```python
from build123d import *

# Parameters (mm, degrees)
SKETCH1_R           = 1.65
SKETCH1_R_2         = 7
BOSS_EXTRUDE1_DEPTH = 3.175


with BuildPart() as part:
    # Sketch1 → Boss-Extrude1 (new body)
    with BuildSketch(Plane(origin=(0, 0, 0), x_dir=(1, 0, 0), z_dir=(0, 1, 0))):
        with BuildLine():
            Line((0, 0), (32, 0))
            Line((32, 0), (32, 27))
            ThreePointArc((32, 27), (16, 43), (0, 27))
            Line((0, 27), (0, 0))
        make_face()
        with Locations(Location((6, 4, 0), (0, 0, 270))):
            Circle(SKETCH1_R, mode=Mode.SUBTRACT)
        with Locations(Location((26, 4, 0), (0, 0, 270))):
            Circle(SKETCH1_R, mode=Mode.SUBTRACT)
        with Locations(Location((16, 27, 0), (0, 0, 270))):
            Circle(SKETCH1_R_2, mode=Mode.SUBTRACT)
    extrude(amount=BOSS_EXTRUDE1_DEPTH)


solid = part.part
```
Check sheet for the modelled part. Datum: model origin and axes. Units: mm. Coordinates: 2 decimals unless noted, no trailing zeros. Loops run counter-clockwise (first coordinate to the right, second up) from the corner with the lowest first, then second, coordinate; pieces in that order, holes last.
1) Sectioned sample at D-D (x = 21). Record the boundary of the cut face in (y, z) (3 decimals), and give its area (3 significant figures).
2) Sectioned sample at B-B (z = -4). Record the boundary of the cut face in (x, y) (3 decimals).
3) Sectioned sample at C-C (y = 0.9). Record the boundary of the cut face in (x, z), and give its area (3 significant figures).
4) Material ranges on probe 1 along X at (y, z) = (0.9, -4); probe 2 along X at (y, z) = (1.35, -27); probe 3 along X at (y, z) = (0.35, -24.5), recorded low to high.
5) Sectioned sample at A-A (x = 6). Record the boundary of the cut face in (y, z) (3 decimals), and give its area (3 significant figures).
6) Release check for a two-part mould opening along X. For faces 1 (the face through (0, 2, -14)), 2 (the face through (16, 2, 0)), 3 (the face through (13.319, 1.565, -20.534)) record: released by +X, released by -X, zero draft, split by the parting line, or undercut.
7) Gauge pin test, flat end, axial feed: pin 1 (2 mm diameter, centred on x = 26, z = -4, fed in from -Y). Record the tip position at first contact, or that the pin passes through.
Check sheet entries:
1. outline: (0, -42.199) - (3.175, -42.199) - (3.175, -31.899) - (0, -31.899) - close; (0, -22.101) - (3.175, -22.101) - (3.175, 0) - (0, 0) - close
1. area: 103 mm2
2. outline: (0, 0) - (4.35, 0) - (4.35, 3.175) - (0, 3.175) - close; (7.65, 0) - (24.35, 0) - (24.35, 3.175) - (7.65, 3.175) - close; (27.65, 0) - (32, 0) - (32, 3.175) - (27.65, 3.175) - close
3. outline: (0, -27) arc R16 ccw to (32, -27) - (32, 0) - (0, 0) - close; hole circle Ø3.3 at (6, -4); hole circle Ø14 at (16, -27); hole circle Ø3.3 at (26, -4)
3. area: 1,100 mm2
4. probe 1: x = 0 to 4.35, 7.65 to 24.35, 27.65 to 32
4. probe 2: x = 0 to 9, 23 to 32
4. probe 3: x = 0 to 9.46, 22.54 to 32
5. outline: (0, -39.49) - (3.175, -39.49) - (3.175, -5.65) - (0, -5.65) - close; (0, -2.35) - (3.175, -2.35) - (3.175, 0) - (0, 0) - close
5. area: 115 mm2
6. face 1: released by -X
6. face 2: zero draft
6. face 3: undercut
7. pin 1: passes through
